from build123d import *

# Parameters (mm, degrees)
F0_R     = 39.37
F1_DEPTH = 88.9
F2_DEPTH = 25.4
F5_DEPTH = 20.32
F5_TAPER = -0.1


with BuildPart() as f1:
    # F0 (on Top) → F1 (new body)
    with BuildSketch(Plane.XY):
        with BuildLine():
            ThreePointArc((168.591448664, 0), (126.4029047972, 64.1394289388), (50.8, 50.8))
            ThreePointArc((50.8, 50.8), (28.891448664, 0), (50.8, -50.8))
            ThreePointArc((50.8, -50.8), (126.4029047972, -64.1394289388), (168.591448664, 0))
        make_face()
        with Locations((98.741448664, 0)):
            Circle(F0_R, mode=Mode.SUBTRACT)
    extrude(amount=F1_DEPTH)

    # F0 (on Top) → F2 (join)
    with BuildSketch(Plane.XY):
        with BuildLine():
            Line((50.8, 50.8), (-50.8, 50.8))
            Line((-50.8, 50.8), (-50.8, -50.8))
            Line((-50.8, -50.8), (50.8, -50.8))
            ThreePointArc((50.8, -50.8), (28.891448664, 0), (50.8, 50.8))
        make_face()
    extrude(amount=F2_DEPTH)

    # F4 (on offset) → F5 (join)
    with BuildSketch(Plane.XZ.offset(10.16)):
        Polygon((28.891448664, 25.4), (28.891448664, 71.12), (-25.4, 25.4), align=None)
    extrude(amount=-F5_DEPTH, taper=F5_TAPER)


solid = f1.part
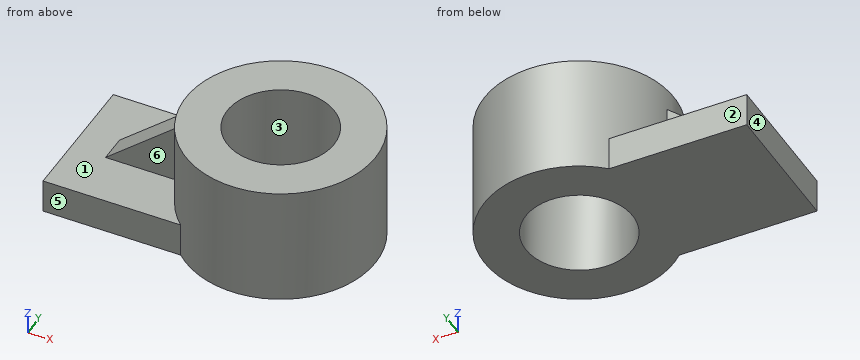
The listing builds one solid part. Answer for the finished solid, in the listing's coordinates (mm). Face numbers are marked on the shaded views. A direction names the side the tool comes from. Coordinates: 2 decimals unless noted, no trailing zeros. Loops run counter-clockwise (first coordinate to the right, second up) from the corner with the lowest first, then second, coordinate; pieces in that order, holes last. Notation, with made-up numbers: M 44.25,83.5 L 77.25,83.5 A21 ccw 77.25,92.5 Z; hole C -1,88 d4. An arc over 180 degrees is marked long. Answer in a Markdown table with one row per item.
1) Find section B-B (x = 83.5). Determine the outline of the cut face in (y, z).
Answers below:
| item | result |
|---|---|
| outline | M -68.17,0 L -36.3,0 L -36.3,88.9 L -68.17,88.9 Z; M 36.3,0 L 68.17,0 L 68.17,88.9 L 36.3,88.9 Z |
2) Find section C-C (z = 21.5). Determine the outline of the cut face in (x, y).
Answers below:
| item | result |
|---|---|
| outline | M -50.8,-50.8 L 50.8,-50.8 A69.85 ccw long 50.8,50.8 L -50.8,50.8 Z; hole C 98.74,0 d78.74 |
3) Find section D-D (y = -25). Determine the outline of the cut face in (x, z).
Answers below:
| item | result |
|---|---|
| outline | M -50.8,0 L 68.33,0 L 68.33,88.9 L 33.52,88.9 L 33.52,25.4 L -50.8,25.4 Z; M 129.16,0 L 163.96,0 L 163.96,88.9 L 129.16,88.9 Z |
4) Given pin 1 (20.5 mm diameter, centred on x = -20, z = 16.5, fed in from -Y); pin 2 (2 mm diameter, centred on y = -47, z = 17, fed in from +X); pin 3 (1 mm diameter, centred on x = 10, z = 58.5, fed in from -Y); pin 4 (4 mm diameter, centred on x = 53.5, z = 76, fed in from +Y), each flat-ended and moving along its own axis, determine where each tip first touches the part or whether it passes through.
Answers below:
| item | result |
|---|---|
| pin 1 | y = -50.8 |
| pin 2 | x = 151.31 |
| pin 3 | through |
| pin 4 | y = 54.86 |
5) Find section A-A (y = 24.5). Determine the outline of the cut face in (x, z).
Answers below:
| item | result |
|---|---|
| outline | M -50.8,0 L 67.92,0 L 67.92,88.9 L 33.33,88.9 L 33.33,25.4 L -50.8,25.4 Z; M 129.56,0 L 164.15,0 L 164.15,88.9 L 129.56,88.9 Z |
6) Determine the mould class of the marked faces 1, 2 and 3 for opening direction Y: released by +Y, released by -Y, zero draft, split by the parting line, or undercut.
Answers below:
| item | result |
|---|---|
| face 1 | zero draft |
| face 2 | released by +Y |
| face 3 | undercut |
7) Which of the six approach directions +Z, -Z, +X, -X, +Y, -Y give full straight-line access (tool end or side, diameter ignored) to the marked faces 4, 5 and 6?
Answers below:
| item | result |
|---|---|
| face 4 | +Z, -Z, -X, +Y, -Y |
| face 5 | +Z, -Z, -X, -Y |
| face 6 | +Z, -X, -Y |
8) Find the intervals of material crossed by probe 1 along Y at (x, z) = (98.5, 56); probe 2 along Y at (x, z) = (28, 4); probe 3 along Z at (x, y) = (9.5, -19), in increasing order.
Answers below:
| item | result |
|---|---|
| probe 1 | -69.85 to -39.37, 39.37 to 69.85 |
| probe 2 | -50.8 to 50.8 |
| probe 3 | 0 to 25.4 |
